Check sheet for the modelled part. Datum: model origin and axes. Units: mm. Face numbers are marked on the shaded views. A direction names the side the tool comes from. Round coordinates to 2 decimals unless told otherwise and drop trailing zeros. Write each loop counter-clockwise with the first axis right and the second up, starting at its lowest first coordinate (ties: lowest second). Pieces come first, ordered by that corner, then holes. Notation, with made-up numbers: (0, 52.5) -> (11, 52.5) arc R27 cw to (11, 78.5) -> close; hole circle Ø10 at (72, -9). An arc over 180 degrees is marked (long way). Put each result on its own line as item: value. Start each with the question number.
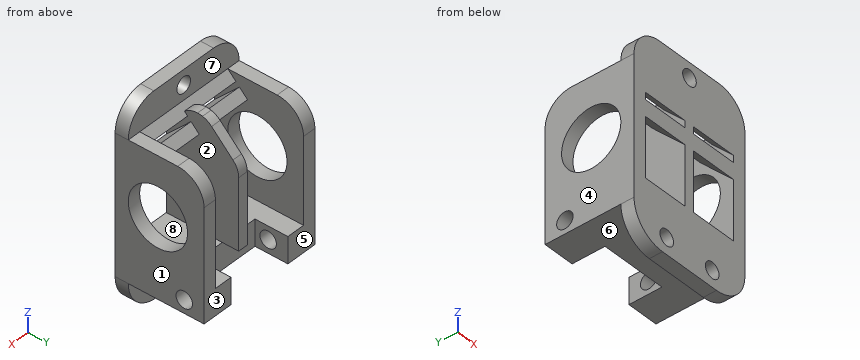
from build123d import *

# Parameters (mm, degrees)
BOSS_EXTRUDE7_DEPTH  = 13.5
SKETCH22_R           = 4.5
CUT_EXTRUDE4_DEPTH   = 41.776818177
SKETCH9_W            = 1.5
SKETCH9_H            = 17
BOSS_EXTRUDE8_DEPTH  = 11
BOSS_EXTRUDE9_DEPTH  = 2
FILLET1_R            = 4
SKETCH11_W           = 10
SKETCH11_H           = 4
CUT_EXTRUDE1_DEPTH   = 5
CHAMFER2_SIZE        = 5
FILLET2_R            = 3
SKETCH12_R           = 1.25
CUT_EXTRUDE2_DEPTH   = 12.5
M2_CLEARANCE_HOLE1_D = 2.4
BOSS_EXTRUDE10_DEPTH = 2
M2_CLEARANCE_HOLE2_D = 2.4
SKETCH20_W           = 15.5
SKETCH20_H           = 8
BOSS_EXTRUDE11_DEPTH = 5.5
CHAMFER3_SIZE        = 5.5
CHAMFER4_START       = -35.400000065
CHAMFER4_DEPTH       = 7
CHAMFER4_START_2     = -26.900000065
CHAMFER4_2_DEPTH     = 7
CHAMFER4_START_3     = -28.400000065
CHAMFER4_3_DEPTH     = 1.5
SKETCH21_W           = 7
SKETCH21_H           = 0.75
CUT_EXTRUDE3_DEPTH   = 46.949966868
LPATTERN1_COUNT      = 2
LPATTERN1_PITCH      = 8.5


with BuildPart() as part:
    # Sketch8 → Boss-Extrude7 (new body)
    with BuildSketch(Plane(origin=(0, 0, 0), x_dir=(1, 0, 0), z_dir=(0, 1, 0))):
        Polygon((-37.400000065, -12.17000001), (-37.400000065, -33.17000001), (-35.400000065, -33.17000001), (-35.400000065, -16.17000001), (-19.900000065, -16.17000001), (-19.900000065, -33.17000001), (-17.900000065, -33.17000001), (-17.900000065, -12.17000001), align=None)
    extrude(amount=BOSS_EXTRUDE7_DEPTH)

    # Sketch22 → Cut-Extrude4 (cut, through all)
    with BuildSketch(Plane.ZY.offset(37.400000065)):
        with Locations((24.17000001, 6.5)):
            Circle(SKETCH22_R)
    extrude(amount=-CUT_EXTRUDE4_DEPTH, mode=Mode.SUBTRACT)

    # Sketch9 → Boss-Extrude8 (add)
    with BuildSketch(Plane(origin=(0, 0, 0), x_dir=(1, 0, 0), z_dir=(0, 1, 0))):
        with Locations((-27.650000065, -24.67000001)):
            Rectangle(SKETCH9_W, SKETCH9_H)
    extrude(amount=BOSS_EXTRUDE8_DEPTH)

    # Sketch10 → Boss-Extrude9 (add)
    with BuildSketch(Plane(origin=(0, 0, 0), x_dir=(1, 0, 0), z_dir=(0, 1, 0))):
        with BuildLine():
            Line((-37.400000065, -30.17000001), (-17.900000065, -30.17000001))
            Line((-17.900000065, -30.17000001), (-17.900000065, -33.17000001))
            ThreePointArc((-17.900000065, -33.17000001), (-19.218019549, -36.351980525), (-22.400000065, -37.67000001))
            Line((-22.400000065, -37.67000001), (-32.900000065, -37.67000001))
            ThreePointArc((-32.900000065, -37.67000001), (-36.08198058, -36.351980525), (-37.400000065, -33.17000001))
            Line((-37.400000065, -33.17000001), (-37.400000065, -30.17000001))
        make_face()
    extrude(amount=BOSS_EXTRUDE9_DEPTH)

    # Fillet1
    fillet1_edges = [part.edges().sort_by_distance(p)[0] for p in [
        (-36.400000065, 13.5, 33.17000001),
        (-18.900000065, 13.5, 33.17000001),
    ]]
    fillet(fillet1_edges, radius=FILLET1_R)

    # Sketch11 → Cut-Extrude1 (cut)
    with BuildSketch(Plane(origin=(0, 13.5, 0), x_dir=(1, 0, 0), z_dir=(0, 1, 0))):
        with Locations((-27.650000065, -14.17000001)):
            Rectangle(SKETCH11_W, SKETCH11_H)
    extrude(amount=-CUT_EXTRUDE1_DEPTH, mode=Mode.SUBTRACT)

    # Chamfer2
    chamfer2_edges = [part.edges().sort_by_distance(p)[0] for p in [
        (-27.650000065, 11, 33.17000001),
    ]]
    chamfer(chamfer2_edges, length=CHAMFER2_SIZE)

    # Fillet2
    fillet2_edges = [part.edges().sort_by_distance(p)[0] for p in [
        (-27.650000065, 11, 28.17000001),
        (-27.650000065, 6, 33.17000001),
    ]]
    fillet(fillet2_edges, radius=FILLET2_R)

    # Sketch12 → Cut-Extrude2 (cut, symmetric)
    with BuildSketch(Plane.ZY.offset(27.650000065)):
        with Locations((14.17000001, 10.5)):
            Circle(SKETCH12_R)
    extrude(amount=CUT_EXTRUDE2_DEPTH, both=True, mode=Mode.SUBTRACT)

    # M2 Clearance Hole1 (through all)
    with Locations(Plane(origin=(-27.650000065, 2, 35.42000001), x_dir=(0, 0, 1), z_dir=(0, 1, 0))):
        with Locations((0, 0)):
            Hole(M2_CLEARANCE_HOLE1_D / 2)

    # Sketch17 → Boss-Extrude10 (add)
    with BuildSketch(Plane(origin=(0, 0, 0), x_dir=(1, 0, 0), z_dir=(0, 1, 0))):
        with BuildLine():
            Line((-32.400000065, -7.17000001), (-22.900000065, -7.17000001))
            ThreePointArc((-22.900000065, -7.17000001), (-19.364466159, -8.634466104), (-17.900000065, -12.17000001))
            Line((-17.900000065, -12.17000001), (-17.900000065, -14.17000001))
            Line((-17.900000065, -14.17000001), (-37.400000065, -14.17000001))
            Line((-37.400000065, -14.17000001), (-37.400000065, -12.17000001))
            ThreePointArc((-37.400000065, -12.17000001), (-35.935533971, -8.634466104), (-32.400000065, -7.17000001))
        make_face()
    extrude(amount=BOSS_EXTRUDE10_DEPTH)

    # M2 Clearance Hole2 (through all)
    with Locations(Plane(origin=(-31.650000065, 2, 9.67000001), x_dir=(0, 0, 1), z_dir=(0, 1, 0))):
        with Locations((0, 0), (0, 8)):
            Hole(M2_CLEARANCE_HOLE2_D / 2)

    # Sketch20 → Boss-Extrude11 (add)
    with BuildSketch(Plane(origin=(0, 0, 0), x_dir=(1, 0, 0), z_dir=(0, 1, 0))):
        with Locations((-27.650000065, -29.17000001)):
            Rectangle(SKETCH20_W, SKETCH20_H)
    extrude(amount=BOSS_EXTRUDE11_DEPTH)

    # Chamfer3
    # the kernel refuses this chamfer: 5.5 mm, written as the material it takes off along each edge
    with BuildSketch(Plane(origin=(-14.255743631, 5.5, 25.17000001), x_dir=(0, 0, 1), z_dir=(-1, 0, 0))) as chamfer3_piece_1_section:
        Polygon((CHAMFER3_SIZE, 0), (0, -CHAMFER3_SIZE), (0, 0), align=None)
    chamfer3_piece_1 = extrude(amount=35.288512868, mode=Mode.PRIVATE)
    chamfer3_piece_1 = split(chamfer3_piece_1, bisect_by=Plane(origin=(-26.900000065, 5.5, 25.17000001), z_dir=(1, 0, 0)), keep=Keep.TOP, mode=Mode.PRIVATE)
    chamfer3_piece_1 = split(chamfer3_piece_1, bisect_by=Plane(origin=(-19.900000065, 5.5, 25.17000001), z_dir=(-1, 0, 0)), keep=Keep.TOP, mode=Mode.PRIVATE)
    add(chamfer3_piece_1, mode=Mode.SUBTRACT)
    with BuildSketch(Plane(origin=(-28.400000065, 5.5, 25.17000001), x_dir=(0, 0, 1), z_dir=(-1, 0, 0)), Plane(origin=(-19.900000065, 5.5, 25.17000001), x_dir=(0, 0, 1), z_dir=(-1, 0, 0))) as chamfer3_piece_2:
        Polygon((CHAMFER3_SIZE, 0), (0, -CHAMFER3_SIZE), (0, 0), align=None)
    extrude(amount=7, mode=Mode.SUBTRACT)
    with BuildSketch(Plane(origin=(-5.755743631, 5.5, 25.17000001), x_dir=(0, 0, 1), z_dir=(-1, 0, 0))) as chamfer3_piece_3_section:
        Polygon((CHAMFER3_SIZE, 0), (0, -CHAMFER3_SIZE), (0, 0), align=None)
    chamfer3_piece_3 = extrude(amount=35.288512868, mode=Mode.PRIVATE)
    chamfer3_piece_3 = split(chamfer3_piece_3, bisect_by=Plane(origin=(-28.400000065, 5.5, 25.17000001), z_dir=(-1, 0, 0)), keep=Keep.TOP, mode=Mode.PRIVATE)
    chamfer3_piece_3 = split(chamfer3_piece_3, bisect_by=Plane(origin=(-35.400000065, 5.5, 25.17000001), z_dir=(1, 0, 0)), keep=Keep.TOP, mode=Mode.PRIVATE)
    add(chamfer3_piece_3, mode=Mode.SUBTRACT)

    # Chamfer4: read off the stored shape, not the designer's step
    # Chamfer4 outline → Chamfer4 (cut)
    with BuildSketch(Plane.YZ.offset(CHAMFER4_START)):
        Polygon((5.5, 30.67000001), (5.5, 33.17000001), (2, 33.17000001), (5, 30.17000001), align=None)
    extrude(amount=CHAMFER4_DEPTH, mode=Mode.SUBTRACT)

    # Chamfer4 2 outline → Chamfer4 2 (cut)
    with BuildSketch(Plane.YZ.offset(CHAMFER4_START_2)):
        Polygon((5.5, 30.67000001), (5.5, 33.17000001), (2, 33.17000001), (5, 30.17000001), align=None)
    extrude(amount=CHAMFER4_2_DEPTH, mode=Mode.SUBTRACT)

    # Chamfer4 3 outline → Chamfer4 3 (cut)
    with BuildSketch(Plane.YZ.offset(CHAMFER4_START_3)):
        with BuildLine():
            ThreePointArc((4.757359313, 33.17000001), (5.131603073, 33.146565415), (5.5, 33.076627748))
            Line((5.5, 33.076627748), (5.5, 33.17000001))
            Line((5.5, 33.17000001), (4.757359313, 33.17000001))
        make_face()
        with BuildLine():
            ThreePointArc((2.760831368, 32.409168642), (3.689067662, 32.973346751), (4.757359313, 33.17000001))
            Line((4.757359313, 33.17000001), (2, 33.17000001))
            Line((2, 33.17000001), (2.760831368, 32.409168642))
        make_face()
    extrude(amount=CHAMFER4_3_DEPTH, mode=Mode.SUBTRACT)

    # Sketch21 → Cut-Extrude3 (cut, through all)
    with BuildSketch(Plane(origin=(0, 17.585000005, 17.585000005), x_dir=(1, 0, 0), z_dir=(0, 0.7071067811865511, 0.707106781186544))):
        with Locations((-31.900000065, -19.919198033)):
            Rectangle(SKETCH21_W, SKETCH21_H)
    cut_extrude3 = extrude(amount=-CUT_EXTRUDE3_DEPTH, mode=Mode.SUBTRACT)

    # LPattern1: Cut-Extrude3 ×2
    with Locations(*[(i * LPATTERN1_PITCH, 0, 0) for i in range(1, LPATTERN1_COUNT)]):
        add(cut_extrude3, mode=Mode.SUBTRACT)


solid = part.part
1. Section check A-A, the plane z = 14.17. Enter the section's corners in (x, y).
2. Section check B-B, the plane x = -27.65. Enter the section's corners in (y, z), then the cut area to 3 significant figures.
3. Gauge pin test, flat ends, axial feed: P1, Ø5, axis at x = -32, y = 7.5, coming from the -Z side; P2, Ø2, axis at x = -23, y = 4.5, coming from the +Z side; P3, Ø2.5, axis at x = -30.5, z = 9.5, coming from the +Y side. Record the tip position at first contact, or that the pin passes through.
4. Section check D-D, the plane x = -23.65. Enter the section's corners in (y, z).
5. Section check C-C, the plane y = 6.5. Enter the section's corners in (x, z), then the cut area to 3 significant figures.
6. Material ranges on L1, parallel to X at y = 4, z = 19.5; L2, parallel to X at y = 1.05, z = 9.67; L3, parallel to Z at x = -24.25, y = 1.5, recorded low to high. Write a range as [from, to].
7. Draft check along X on the marked faces 1, 2 and 3. Enter one of: released by +X, released by -X, zero draft, split by the parting line, or undercut.
8. Access from +Z, -Z, +X, -X, +Y, -Y to the whole of each face (thin tool, end or side, straight path). Record for the marked faces 4, 5, 6, 7 and 8.
Reply:
1. outline: (-37.4, 0) -> (-17.9, 0) -> (-17.9, 9.25) -> (-22.65, 9.25) -> (-22.65, 8.5) -> (-32.65, 8.5) -> (-32.65, 9.25) -> (-37.4, 9.25) -> close; (-37.4, 11.75) -> (-32.65, 11.75) -> (-32.65, 13.5) -> (-37.4, 13.5) -> close; (-22.65, 11.75) -> (-17.9, 11.75) -> (-17.9, 13.5) -> (-22.65, 13.5) -> close
2. outline: (0, 7.17) -> (2, 7.17) -> (2, 12.17) -> (8.5, 12.17) -> (8.5, 16.17) -> (11, 16.17) -> (11, 26.93) arc R3 ccw to (10.12, 29.05) -> (6.88, 32.29) arc R3 ccw to (2.76, 32.41) -> (2, 33.17) -> (2, 34.22) -> (0, 34.22) -> close; (0, 36.62) -> (2, 36.62) -> (2, 37.67) -> (0, 37.67) -> close
2. area: 222 mm2
3. P1: stops at z = 12.17
3. P2: stops at z = 31.4
3. P3: stops at y = 2
4. outline: (0, 7.17) -> (2, 7.17) -> (2, 8.47) -> (0, 8.47) -> close; (0, 10.87) -> (2, 10.87) -> (2, 12.17) -> (8.5, 12.17) -> (8.5, 16.17) -> (0, 16.17) -> close; (0, 25.17) -> (5, 30.17) -> (3.77, 31.4) -> (0, 27.64) -> close; (0, 28.7) -> (3.23, 31.94) -> (2, 33.17) -> (2, 37.67) -> (0, 37.67) -> close
5. outline: (-37.4, 12.17) -> (-17.9, 12.17) -> (-17.9, 19.67) -> (-19.9, 19.67) -> (-19.9, 16.17) -> (-26.9, 16.17) -> (-26.9, 32.61) -> (-28.4, 32.61) -> (-28.4, 16.17) -> (-35.4, 16.17) -> (-35.4, 19.67) -> (-37.4, 19.67) -> close; (-37.4, 28.67) -> (-35.4, 28.67) -> (-35.4, 33.17) -> (-37.4, 33.17) -> close; (-19.9, 28.67) -> (-17.9, 28.67) -> (-17.9, 33.17) -> (-19.9, 33.17) -> close
5. area: 135 mm2
6. L1: x = [-37.4, -35.4], [-28.4, -26.9], [-19.9, -17.9]
6. L2: x = [-36.73, -32.85], [-30.45, -24.85], [-22.45, -18.57]
6. L3: z = [7.17, 8.63], [10.71, 16.17], [26.67, 29.14], [30.2, 37.67]
7. face 1: released by +X
7. face 2: undercut
7. face 3: zero draft
8. face 4: +Z, -Z, -X, +Y, -Y
8. face 5: +Z, -Z, +X, -X, +Y
8. face 6: -Z, +X, -X, +Y
8. face 7: +Z, +X, -X, +Y
8. face 8: +Y, -Y
